Can you work these out from the model? Positions are in its coordinate system, mm. Round coordinates to 2 decimals unless told otherwise and drop trailing zeros. Write each loop counter-clockwise with the first axis right and the second up, starting at its lowest first coordinate (ties: lowest second). Pieces come first, ordered by that corner, then holes.
Q1. If we section it at B-B (z = 9.5): Please give me the cut outline in (x, y).
Q2. We'd pull the mould along Z, two halves only. Please class faces 1 (the flat face through (-42, 151, 0)), 2 (the cylindrical face through (-0.92, 22.39, 41.99)), 3 (the cylindrical face through (-44, 223, 0)): +Z half, -Z half, draft (parallel to the pull), parting line (faces both ways), or undercut.
Q3. If we section it at D-D (x = 0): Please give me the cut outline in (y, z), plus the area to 3 significant figures.
Q4. I'm going to push flat-ended pins straight in: pin 1 Ø3.5 at (y, z) = (220, 0) entering from +X; pin 2 Ø2 at (x, y) = (-44, 210) entering from +Z. Where does each tip first touch, or does it pass through?
Q5. If we section it at C-C (y = 220): Please give me the cut outline in (x, z), plus the area to 3 significant figures.
Q6. If we section it at A-A (y = 135): Please give me the cut outline in (x, z).
Q7. Please list where these lines run through material, in increasing order: line 1 along Z through (x, y) = (43, 220); line 2 along Y through (x, z) = (-43.7, 0); line 3 along X through (y, z) = (178.5, 5).
from build123d import *

# Parameters (mm, degrees)
EXTRUDE_1_DEPTH     = 30
SKETCH_4_W          = 4
SKETCH_4_H          = 24
EXTRUDE_3_DEPTH     = 260
SKETCH_7_W          = 149.597155604
SKETCH_7_H          = 115.941502163
CUT_EXTRUDE_3_DEPTH = 59
SKETCH_9_R          = 3
CUT_EXTRUDE_5_DEPTH = 93
SKETCH_10_R         = 50
SKETCH_10_R_2       = 46
CUT_EXTRUDE_6_DEPTH = 15


with BuildPart() as part:
    # 草图1 → 凸台-拉伸1 (new body)
    with BuildSketch(Plane(origin=(0, 0, 0), x_dir=(1, 0, 0), z_dir=(0, 1, 0))):
        with BuildLine():
            Line((-46, 0), (-46, 12))
            Line((-46, 12), (-42, 12))
            Line((-42, 12), (-42, 0))
            ThreePointArc((-42, 0), (0, -42), (42, 0))
            Line((42, 0), (42, 12))
            Line((42, 12), (46, 12))
            Line((46, 12), (46, 0))
            ThreePointArc((46, 0), (0, -46), (-46, 0))
        make_face()
    extrude(amount=EXTRUDE_1_DEPTH)

    # 草图4 → 凸台-拉伸3 (add)
    with BuildSketch(Plane(origin=(0, 30, 0), x_dir=(1, 0, 0), z_dir=(0, 1, 0))):
        with Locations((44, 0)):
            Rectangle(SKETCH_4_W, SKETCH_4_H)
        with Locations((-44, 0)):
            Rectangle(SKETCH_4_W, SKETCH_4_H)
    extrude(amount=EXTRUDE_3_DEPTH)

    # 草图7 → 切除-拉伸3 (cut, through all)
    with BuildSketch(Plane(origin=(0, 0, -12), x_dir=(-1, 0, 0), z_dir=(0, 0, -1))):
        with Locations((8.175952602, -42.970751082)):
            Rectangle(SKETCH_7_W, SKETCH_7_H)
    extrude(amount=-CUT_EXTRUDE_3_DEPTH, mode=Mode.SUBTRACT)

    # 草图9 → 切除-拉伸5 (cut, through all)
    with BuildSketch(Plane(origin=(46, 0, 0), x_dir=(0, 0, -1), z_dir=(1, 0, 0))):
        with Locations((0, 220)):
            Circle(SKETCH_9_R)
    extrude(amount=-CUT_EXTRUDE_5_DEPTH, mode=Mode.SUBTRACT)

    # 草图10 → 切除-拉伸6 (cut)
    with BuildSketch(Plane.XZ.offset(-15)):
        Circle(SKETCH_10_R)
        Circle(SKETCH_10_R_2, mode=Mode.SUBTRACT)
    extrude(amount=-CUT_EXTRUDE_6_DEPTH, mode=Mode.SUBTRACT)


solid = part.part
A:
1. outline: (-46, 30) - (-45.01, 30) - (-45.01, 15) - (-40.91, 15) - (-40.91, 30) - (-42, 30) - (-42, 290) - (-46, 290) - close; (40.91, 15) - (45.01, 15) - (45.01, 30) - (46, 30) - (46, 290) - (42, 290) - (42, 30) - (40.91, 30) - close
2. face 1: draft
2. face 2: -Z half
2. face 3: undercut
3. outline: (15, 42) - (30, 42) - (30, 46) - (15, 46) - close
3. area: 60.0 mm2
4. pin 1: passes through
4. pin 2: stops at z = 12
5. outline: (-46, -12) - (-42, -12) - (-42, -3) - (-46, -3) - close; (-46, 3) - (-42, 3) - (-42, 12) - (-46, 12) - close; (42, -12) - (46, -12) - (46, -3) - (42, -3) - close; (42, 3) - (46, 3) - (46, 12) - (42, 12) - close
5. area: 144 mm2
6. outline: (-46, -12) - (-42, -12) - (-42, 12) - (-46, 12) - close; (42, -12) - (46, -12) - (46, 12) - (42, 12) - close
7. line 1: z = -12 to -3, 3 to 12
7. line 2: y = 15 to 217, 223 to 290
7. line 3: x = -46 to -42, 42 to 46
